Geometry: final body of the model. Coordinates: model frame, mm. Face numbers are marked on the shaded views. A direction names the side the tool comes from. Coordinates: 2 decimals unless noted, no trailing zeros. Loops run counter-clockwise (first coordinate to the right, second up) from the corner with the lowest first, then second, coordinate; pieces in that order, holes last. Notation, with made-up numbers: (27, 59) - (63, 59) arc R38 ccw to (63, 98) - close; hole circle Ø11 at (81.25, -27.5). An arc over 180 degrees is marked (long way). Return JSON: item names as keys, results as strings.
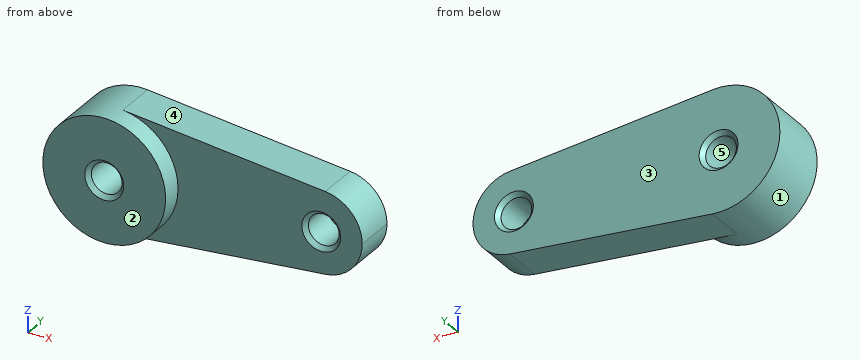
from build123d import *

# Parameters (mm, degrees)
F1_R     = 9.525
F2_DEPTH = 25.4
F0_R     = 38.1
F0_R_2   = 9.525
F3_DEPTH = 38.1
F4_SIZE  = 2.54


with BuildPart() as f2:
    # F1 (on face) → F2 (new body)
    with BuildSketch(Plane.XZ):
        with BuildLine():
            ThreePointArc((-13.4022655529, 0), (-23.2465491404, 25.5582567875), (-47.6922650288, 37.9090213011))
            ThreePointArc((-47.6922650288, 37.9090213011), (-89.6022655529, 2.206e-07), (-47.6922654678, -37.9090213452))
            ThreePointArc((-47.6922654678, -37.9090213452), (-23.2465492884, -25.5582569511), (-13.4022655529, 0))
        make_face()
        with Locations((-51.5022655529, 0)):
            Circle(F1_R, mode=Mode.SUBTRACT)
        with BuildLine():
            Line((78.0377345258, 25.2726808946), (-47.6922650288, 37.9090213011))
            ThreePointArc((-47.6922650288, 37.9090213011), (-23.2465491404, 25.5582567875), (-13.4022655529, 0))
            ThreePointArc((-13.4022655529, 0), (-23.2465492884, -25.5582569511), (-47.6922654678, -37.9090213452))
            Line((-47.6922654678, -37.9090213452), (78.0377338702, -25.2726809605))
            ThreePointArc((78.0377338702, -25.2726809605), (50.0977344471, 3.295e-07), (78.0377345258, 25.2726808946))
        make_face()
        with BuildLine():
            ThreePointArc((100.8977344471, 0), (94.3348786309, 17.0388379592), (78.0377345258, 25.2726808946))
            ThreePointArc((78.0377345258, 25.2726808946), (50.0977344471, 3.295e-07), (78.0377338702, -25.2726809605))
            ThreePointArc((78.0377338702, -25.2726809605), (94.3348784099, -17.0388382036), (100.8977344471, 0))
        make_face()
        with Locations((75.4977344471, 0)):
            Circle(F1_R, mode=Mode.SUBTRACT)
    extrude(amount=F2_DEPTH)

    # F0 (on Front) → F3 (join)
    with BuildSketch(Plane.XZ):
        with Locations((-51.5022655529, 0)):
            Circle(F0_R)
        with Locations((-51.5022655529, 0)):
            Circle(F0_R_2, mode=Mode.SUBTRACT)
    extrude(amount=F3_DEPTH)

    # F4
    f4_edges = [f2.edges().sort_by_distance(p)[0] for p in [
        (85.022734, -12.7, 0),
        (65.972734, 0, 0),
        (65.972734, -25.4, 0),
        (-61.027266, 0, 0),
        (-41.977266, -19.05, 0),
        (-61.027266, -38.1, 0),
    ]]
    chamfer(f4_edges, length=F4_SIZE)


solid = f2.part
Item 1: Section query C-C, the plane z = -30. Return loops of the section in (x, y).
Worked out:
{"outline": "(-74.99, -38.1) - (-28.02, -38.1) - (-28.02, -25.4) - (31, -25.4) - (31, 0) - (-74.99, 0) - close"}
Item 2: Ray query, probe 1 along X at (y, z) = (-12.5, 1); probe 2 along Y at (x, z) = (-12.5, 14.5); probe 3 along X at (y, z) = (-36, -7.5). Return the intervals inside material, ascending. Write a range as from..to.
Worked out:
{"probe 1": "-89.59..-60.97, -42.03..66.03, 84.97..100.88", "probe 2": "-25.4..0", "probe 3": "-88.86..-58.06, -44.94..-14.15"}
Item 3: First-contact query: pin 1 Ø6 at (y, z) = (-17, 14.5) entering from -X; pin 2 Ø25 at (x, z) = (75.5, 0) entering from -Y; pin 3 Ø5 at (y, z) = (-5.5, -11.5) entering from -X. Flat tips, straight axial feed; report the tip coordinate or a pass-through.
Worked out:
{"pin 1": "x = -87.83", "pin 2": "y = -25.4", "pin 3": "x = -88.52"}
Item 4: Section query D-D, the plane x = 14. Return loops of the section in (y, z).
Worked out:
{"outline": "(-25.4, -31.71) - (0, -31.71) - (0, 31.71) - (-25.4, 31.71) - close"}
Item 5: Section query B-B, the plane y = -29. Return loops of the section in (x, z) (3 decimals).
Worked out:
{"outline": "circle Ø76.2 at (-51.502, 0); hole circle Ø19.05 at (-51.502, 0)"}
Item 6: Section query A-A, the plane y = -19. Return loops of the section in (x, z) (3 decimals).
Worked out:
{"outline": "(-47.692, -37.909) - (78.038, -25.273) arc R25.4 ccw to (78.038, 25.273) - (-47.692, 37.909) arc R38.1 ccw (long way) to start; hole circle Ø19.05 at (-51.502, 0); hole circle Ø19.05 at (75.498, 0)"}
Item 7: Reachability of the marked faces 1 and 2 from +Z, -Z, +X, -X, +Y, -Y: full face, straight path, thin tool, end or side. Return the list, or none.
Worked out:
{"face 1": "-Y", "face 2": "+Z, -Z, +X, -X, -Y"}
Item 8: Mould query, pull axis Z, two halves, no side actions, for the marked faces 3, 4 and 5. Classes: +Z half, -Z half, draft (parallel to the pull), parting line (faces both ways), or undercut.
Worked out:
{"face 3": "draft", "face 4": "+Z half", "face 5": "undercut"}
